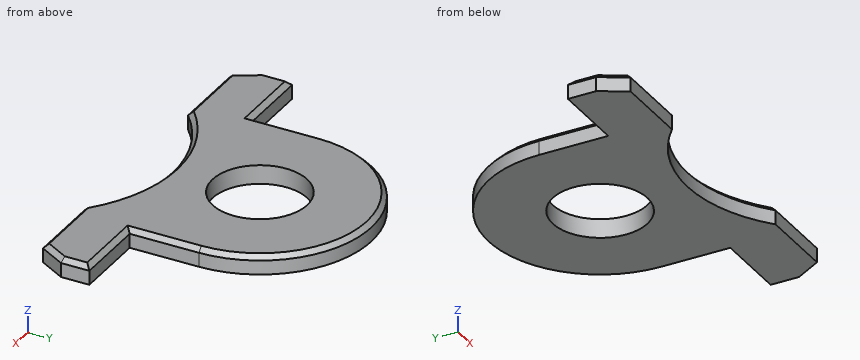
Solid Edge part; units mm, degrees
sketch "Sketch1" plane through (0, 0, 0) normal (0, 0, 1) x (1, 0, 0)
  arc A0 (-9.9816, -10.6836) -> (10.0488, -10.6836) centre (0.0336, -21.8503) cw
  line L0 (10.0488, -10.6836) -> (18.0488, -10.6836)
  line L1 (18.0488, -10.6836) -> (19.6336, -7.914)
  line L2 (19.6336, -4.914) -> (19.6336, -7.914)
  line L3 (11.8299, -4.914) -> (19.6336, -4.914)
  line L4 (11.8299, 2.3997) -> (11.8299, -4.914)
  arc A1 (-11.7627, 2.3997) -> (11.8299, 2.3997) centre (0.0336, 2.3997) cw
  line L5 (-11.7627, 2.3997) -> (-11.7627, -4.914)
  line L6 (-19.5664, -4.914) -> (-11.7627, -4.914)
  line L7 (-19.5664, -4.914) -> (-19.5664, -7.914)
  line L8 (-17.9816, -10.6836) -> (-19.5664, -7.914)
  line L9 (-9.9816, -10.6836) -> (-17.9816, -10.6836)
  dimension "D1" = 19.6336
  dimension "D2" = 10.0488
extrude "Protrusion1" add sketch "Sketch1" along normal blind 2
chamfer "Fase_1" distance 0.5 angle 45 12 edges at (14.0488, -10.6836, 2) (0.0336, -6.8503, 2) (-13.9816, -10.6836, 2) (-18.774, -9.2988, 2) (-19.5664, -6.414, 2) (-15.6646, -4.914, 2) (-11.7627, -1.2572, 2) (0.0336, 14.196, 2) (11.8299, -1.2572, 2) (15.7317, -4.914, 2) (19.6336, -6.414, 2) (18.8412, -9.2988, 2)
sketch "Sketch2" plane through (0.0336, 1.7562, 2) normal (0, 0, 1) x (1, 0, 0)
  circle A0 centre (0, 0.6435) radius 5
extrude "Cutout1" cut sketch "Sketch2" against normal through all
Geometry: final body of the model. Coordinates: model frame, mm. Round coordinates to 2 decimals unless told otherwise and drop trailing zeros. Order: outer loops, then holes, each group sorted by start corner. A loop starts at its lowest first (then second) coordinate and runs counter-clockwise, first axis right, second up. Notation, with made-up numbers: (52, -38.75) -> (69, -38.75) arc R30 ccw to (69, -16.75) -> close; hole circle Ø4 at (29.5, 13.5). An arc over 180 degrees is marked (long way). Use one line per item in the form item = value. Start each with the question number.
1. Line query: probe 1 along Y at (x, z) = (16, 0.2); probe 2 along X at (y, z) = (-3, 0.5); probe 3 along Y at (x, z) = (4.5, 1.7). Output: solid intervals per line, ascending.
2. Cut plane C-C (y = 1). Return the cut outline in (x, z), then the cut area to 3 significant figures.
3. Pin query (flat end, axial travel): pin 1 Ø0.8 at (x, z) = (-14, 1) entering from +Y; pin 2 Ø0.8 at (y, z) = (-1.5, 1) entering from -X. Return the tip coordinate at first contact, or that it passes through.
4. Cut plane B-B (x = -14). Return the cut outline in (y, z).
Solution:
q1.probe_1 = -10.68 to -4.91
q1.probe_2 = -11.76 to 11.83
q1.probe_3 = -7.32 to 0.15, 4.65 to 13.1
q2.outline = (-11.76, 0) -> (-4.77, 0) -> (-4.77, 2) -> (-11.26, 2) -> (-11.76, 1.5) -> close; (4.83, 0) -> (11.83, 0) -> (11.83, 1.5) -> (11.33, 2) -> (4.83, 2) -> close
q2.area = 27.7 mm^2
q3.pin_1 = -4.91
q3.pin_2 = -11.76
q4.outline = (-10.68, 0) -> (-4.91, 0) -> (-4.91, 1.5) -> (-5.41, 2) -> (-10.18, 2) -> (-10.68, 1.5) -> close
